Read the model definition and answer for the solid it produces. Units are mm, in the model's axes. Face numbers are marked on the shaded views. A direction names the side the tool comes from. Coordinates: 2 decimals unless noted, no trailing zeros. Order: outer loops, then holes, each group sorted by start corner. A loop starts at its lowest first (then second) coordinate and runs counter-clockwise, first axis right, second up. Notation, with made-up numbers: (42.25, 81) -> (53.25, 81) arc R10 cw to (53.25, 99) -> close; hole circle Ø4 at (-40, 20.25). An arc over 180 degrees is marked (long way). Use CSV: the item, a comma, the result in double quotes.
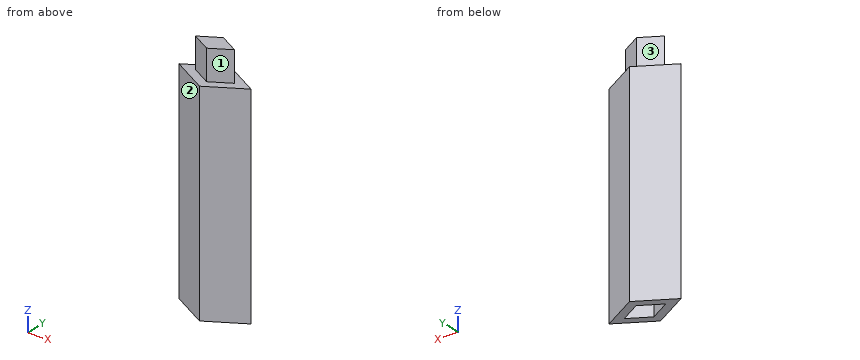
```python
from build123d import *

# Parameters (mm, degrees)
F1_DEPTH = 50.8
F3_DEPTH = 127
F5_DEPTH = 25.4


with BuildPart() as f1:
    # F0 (on Top) → F1 (new body)
    with BuildSketch(Plane.XY):
        Polygon((-30.099, 0), (-17.3265462716, 0), (0, 9.9280379058), (0, 17.2466), align=None)
        Polygon((0, 17.2466), (0, 9.9280379058), (17.3265462716, 0), (30.099, 0), align=None)
        Polygon((30.099, 0), (17.3265462716, 0), (0, -9.9280379058), (0, -17.2466), align=None)
        Polygon((0, -9.9280379058), (-17.3265462716, 0), (-30.099, 0), (0, -17.2466), align=None)
    extrude(amount=F1_DEPTH)

    # F2 (on face) → F3 (join)
    with BuildSketch(Plane.XY.offset(50.8)):
        Polygon((-30.099, 0), (0, -17.2466), (30.099, 0), (0, 17.2466), align=None)
        Polygon((0, -9.9280379058), (-17.3265462716, 0), (0, 9.9280379058), (17.3265462716, 0), align=None, mode=Mode.SUBTRACT)
        Polygon((0, 9.9280379058), (-17.3265462716, 0), (0, -9.9280379058), (17.3265462716, 0), align=None)
    extrude(amount=F3_DEPTH)

    # F4 (on face) → F5 (join)
    with BuildSketch(Plane.XY.offset(177.8)):
        Polygon((0, 9.3425529383), (-16.3047499733, 0), (0, -9.3425529383), (16.3047499733, 0), align=None)
    extrude(amount=F5_DEPTH)


solid = f1.part
```
Item 1: Each of these flat-tipped pins is pushed along its axis until it touches: P1, Ø2, axis at y = 10.5, z = 123, coming from the -X side; P2, Ø1, axis at x = 19, z = 153, coming from the -Y side; P3, Ø4, axis at x = -5, z = 177.5, coming from the +Y side. Where does it stop, or does it pass through?
Return value:
P1,"stops at x = -13.52"
P2,"stops at y = -6.65"
P3,"stops at y = 15.53"
Item 2: A tool of negligible diameter and unlimited length cuts with its end or side. For the marked faces 1, 2 and 3, from which of +Z, -Z, +X, -X, +Y, -Y can it reach the whole face along a straight path? Write none if from no direction.
Return value:
face 1,"+Z, +X, -Y"
face 2,"+Z, -Z, -X, -Y"
face 3,"+Z, -X, +Y"
Item 3: Find section A-A, the plane z = 32.5. Give the vertices of the cut face in (x, y).
Return value:
outline,"(-30.1, 0) -> (0, -17.25) -> (30.1, 0) -> (0, 17.25) -> close; hole (-17.33, 0) -> (0, -9.93) -> (17.33, 0) -> (0, 9.93) -> close"
Item 4: Find section D-D, the plane z = 120. Give the vertices of the cut face in (x, y).
Return value:
outline,"(-30.1, 0) -> (0, -17.25) -> (30.1, 0) -> (0, 17.25) -> close"
Item 5: Find section B-B, the plane x = -4. Give the vertices of the cut face in (y, z), then the cut area to 3 significant figures.
Return value:
outline,"(-14.95, 0) -> (-7.64, 0) -> (-7.64, 50.8) -> (7.64, 50.8) -> (7.64, 0) -> (14.95, 0) -> (14.95, 177.8) -> (7.05, 177.8) -> (7.05, 203.2) -> (-7.05, 203.2) -> (-7.05, 177.8) -> (-14.95, 177.8) -> close"
area,"4,900 mm^2"
Item 6: Find section C-C, the plane y = 2. Give the vertices of the cut face in (x, z).
Return value:
outline,"(-26.61, 0) -> (-13.84, 0) -> (-13.84, 50.8) -> (13.84, 50.8) -> (13.84, 0) -> (26.61, 0) -> (26.61, 177.8) -> (12.81, 177.8) -> (12.81, 203.2) -> (-12.81, 203.2) -> (-12.81, 177.8) -> (-26.61, 177.8) -> close"
Item 7: Straight lines are drawn through the part: line 1 along Z through (x, y) = (1, -11.5); line 2 along X through (y, z) = (4, 184); line 3 along Z through (x, y) = (-3, 8). For each, find the intervals that lie inside material, in ascending order.
Return value:
line 1,"z = 0 to 177.8"
line 2,"x = -9.32 to 9.32"
line 3,"z = 50.8 to 177.8"
